Source: CAD feature listing. Evaluate the final solid. Frame: model axes, mm. Face numbers are marked on the shaded views. A direction names the side the tool comes from. Give positions to 0.01 mm unless a question says otherwise; leave off trailing zeros. Use one line per item in the form item = value. Start each with the question number.
(1) Draft query along X for the marked faces 1, 2 and 3. Return one class per face: pulls with the +X half, pulls with the -X half, needs draft (parallel to the pull), parting line crosses it, or undercut.
(2) Material intervals for line 1 along Y through (x, z) = (3, 14.25); line 2 along Z through (x, y) = (15, -34); line 3 along X through (y, z) = (2, 21), sorted ascending. Write a range as from..to.
(3) Set-up query: the marked faces 4 and 5. Return all of +Z, -Z, +X, -X, +Y, -Y with unobstructed straight access to the full face (end or side cutting, diameter ignored); none if empty.
(4) Cut plane A-A, the plane z = 3. Count the separate pieces of the cut face and the enclosed holes in it, and give its area (3 significant figures).
(5) First-contact query: P1, Ø3, axis at x = 9.88, y = -30.61, coming from the -Z side; P2, Ø12, axis at y = 15, z = 14.5, coming from the +X side; P3, Ø2, axis at y = 11, z = 13, coming from the +X side; P4, Ø2, axis at x = 5, z = 6.5, coming from the +Y side. Flat tips, straight axial feed; report the tip coordinate or a pass-through.
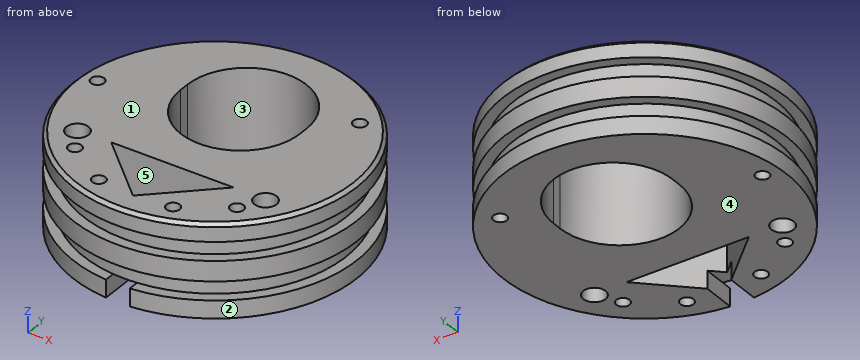
Autodesk Inventor part; units mm, degrees
ref_plane "Work Plane1" through (0, 0, 21.59) normal (0, 0, 1) x (1, 0, 0)
ref_plane "Work Plane2" through (0, 0, 6.35) normal (0, 0, -1) x (-1, 0, 0)
ref_plane "Work Plane4" through (-16.2938, -35.56, 1.651) normal (0, -1, 0) x (1, 0, 0)
sketch "Sketch1" plane through (0, 0, 0) normal (0, 0, 1) x (1, 0, 0)
  circle A0 centre (0, 0) radius 37.7444
  dimension "d0" = 75.4888
extrude "Extrusion1" add sketch "Sketch1" along normal blind 27.94
ref_plane "Work Plane1" through (0, 0, 21.59) normal (0, 0, 1) x (1, 0, 0)
sketch "Sketch2" plane through (0, 0, 21.59) normal (0, 0, 1) x (1, 0, 0)
  circle A0 centre (0, 0) radius 34.9504
  circle A1 centre (0, 0) radius 37.7444
  dimension "d4" = 2.794
extrude "Extrusion2" cut sketch "Sketch2" against normal blind 4.953
ref_plane "Work Plane2" through (0, 0, 6.35) normal (0, 0, -1) x (-1, 0, 0)
sketch "Sketch3" plane through (0, 0, 6.35) normal (0, 0, -1) x (-1, 0, 0)
  circle A0 centre (0, 0) radius 34.9504
  circle A1 centre (0, 0) radius 37.7444
  dimension "d8" = 2.794
extrude "Extrusion3" cut sketch "Sketch3" against normal blind 4.953
sketch "Sketch4" plane through (0, 0, 0) normal (0, 0, -1) x (-1, 0, 0)
  circle A0 centre (0, 0) radius 31.7754
  line L0 (-29.1271, -12.7) -> (29.1271, -12.7)
  line L1 (-19.685, -12.7) -> (-19.685, 24.9435)
  line L2 (19.685, -12.7) -> (19.685, 24.9435)
  line L3 (0, -52.8422) -> (0, 52.8422)
  circle A1 centre (0, 0) radius 37.7444
  line L4 (52.8422, 0) -> (-52.8422, 0)
  dimension "d11" = 39.37
  dimension "d12" = 5.969
  dimension "d25" = 12.7
extrude "Extrusion4" [suppressed]
sketch "Sketch5" plane through (0, 0, 27.94) normal (0, 0, 1) x (1, 0, 0)
  circle A0 centre (24.257, 20.828) radius 1.778
  circle A1 centre (-21.59, -22.86) radius 1.778
  circle A2 centre (21.59, -22.86) radius 1.778
  line L0 (0, -52.8422) -> (0, 52.8422)
  line L1 (-52.8422, 0) -> (52.8422, 0)
  circle A3 centre (-33.02, 2.54) radius 1.778
  point P0 (0, 0)
  dimension "d16" = 3.556
  dimension "d17" = 3.556
  dimension "d18" = 3.556
  dimension "d19" = 20.828
  dimension "d20" = 24.257
  dimension "d21" = 22.86
  dimension "d22" = 21.59
  dimension "d64" = 3.556
  dimension "d65" = 2.54
  dimension "d66" = 33.02
extrude "Extrusion5" cut sketch "Sketch5" against normal through all
sketch "Sketch6" plane through (0, 0, 27.94) normal (0, 0, 1) x (1, 0, 0)
  circle A0 centre (21.59, -22.86) radius 1.778
  circle A1 centre (24.257, 20.828) radius 1.778
  circle A2 centre (-21.59, -22.86) radius 1.778
  circle A3 centre (0, 0) radius 37.7444
  circle A4 centre (-21.59, -22.86) radius 1.778
  circle A5 centre (-21.59, -22.86) radius 8.255
  circle A6 centre (21.59, -22.86) radius 8.255
  line L0 (-16.3153, -16.51) -> (26.8647, -16.51)
  circle A7 centre (0, 0) radius 34.9504
  circle A8 centre (0, 0) radius 31.7754
  line L1 (0, -31.7754) -> (-16.2938, -16.51)
  line L2 (0, -31.7754) -> (16.2938, -16.51)
  dimension "d26" = 16.51
  dimension "d27" = 16.51
extrude "Extrusion6" cut sketch "Sketch6" against normal through all contours L2 L1 L0
fillet "Fillet1" [suppressed]
chamfer "Chamfer1" distance 2.54 angle 45 1 edges at (-37.7444, 0, 27.94)
sketch "Sketch9" plane through (0, 0, 27.94) normal (0, 0, 1) x (1, 0, 0)
  circle A0 centre (-9.8806, -30.607) radius 1.778
  circle A1 centre (9.8806, -30.607) radius 1.778
  line L0 (-52.8422, 0) -> (52.8422, 0)
  line L1 (0, -52.8422) -> (0, 52.8422)
  line L2 (-14.9225, -28.448) -> (14.9225, -28.448)
  line L3 (14.9225, -28.448) -> (14.9225, -34.163)
  line L4 (14.9225, -34.163) -> (-14.9225, -34.163)
  line L5 (-14.9225, -34.163) -> (-14.9225, -28.448)
  point P0 (0, 0)
  dimension "d45" = 3.556
  dimension "d46" = 3.556
  dimension "d47" = 19.7612
  dimension "d48" = 29.845
  dimension "d49" = 5.715
  dimension "d50" = 3.556
  dimension "d51" = 34.163
extrude "Extrusion9" cut sketch "Sketch9" against normal through all contours A0 | A1
sketch "Sketch11" plane through (0, 0, 0) normal (0, 0, -1) x (-1, 0, 0)
  circle A0 centre (-9.8806, -30.607) radius 1.778
  circle A1 centre (9.8806, -30.607) radius 1.778
  line L0 (16.2938, -16.51) -> (0, -31.7754)
  line L1 (0, -31.7754) -> (-16.2938, -16.51)
  line L2 (-16.2938, -16.51) -> (16.2938, -16.51)
  circle A2 centre (-21.59, -22.86) radius 1.778
  circle A3 centre (-24.257, 20.828) radius 1.778
  circle A4 centre (21.59, -22.86) radius 1.778
  circle A5 centre (0, 0) radius 37.7444
extrude "Extrusion10" cut sketch "Sketch11" against normal blind 1.651
sketch "Sketch12" plane through (0, 0, 27.94) normal (0, 0, 1) x (1, 0, 0)
  circle A0 centre (9.8806, -30.607) radius 1.778
  circle A1 centre (-9.8806, -30.607) radius 1.778
  circle A2 centre (-21.59, -22.86) radius 1.778
  circle A3 centre (24.257, 20.828) radius 1.778
  circle A4 centre (21.59, -22.86) radius 1.778
  line L0 (0, -31.7754) -> (-16.2938, -16.51)
  line L1 (-16.2938, -16.51) -> (16.2938, -16.51)
  line L2 (16.2938, -16.51) -> (0, -31.7754)
  circle A5 centre (0, 0) radius 35.2044
  circle A6 centre (0, 0) radius 37.7444
extrude "Extrusion11" cut sketch "Sketch12" against normal blind 1.651 contours A0 | A1 | A2 | A3 | A4 | L0 L1 L2 | A5 | A6
ref_plane "Work Plane4" through (-16.2938, -35.56, 1.651) normal (0, -1, 0) x (1, 0, 0)
sketch "Sketch13" plane through (-16.2938, -35.56, 1.651) normal (0, -1, 0) x (1, 0, 0)
  line L0 (16.2938, -7.239) -> (16.2938, 31.877)
  line L1 (-36.5483, -1.651) -> (69.136, -1.651)
  line L2 (8.1912, 24.638) -> (8.1912, 0)
  line L3 (54.0382, 0) -> (-21.4506, 0)
  line L4 (-21.4506, 4.699) -> (54.0382, 4.699)
  line L5 (39.6618, 24.638) -> (39.6618, 0)
  line L6 (51.2442, 4.699) -> (-18.6566, 4.699)
  line L7 (-2.049, 0) -> (34.6366, 0)
  line L8 (13.1188, 4.699) -> (19.4688, 4.699)
  line L9 (19.4688, 4.699) -> (19.4688, 0)
  line L10 (19.4688, 0) -> (13.1188, 0)
  line L11 (13.1188, 0) -> (13.1188, 4.699)
  point P0 (16.2938, -1.651)
  point P1 (13.1188, 0)
  point P2 (19.4688, 0)
  dimension "d61" = 6.35
extrude "Extrusion12" cut sketch "Sketch13" against normal mid plane 25.4 contours L3 L11 L4 L0 | L0 L4 L9 L3
sketch "Sketch14" plane through (0, 0, 1.651) normal (0, 0, -1) x (-1, 0, 0)
  circle A0 centre (-25.0506, -16.8477) radius 2.9591
  circle A1 centre (25.0506, -16.8477) radius 2.9591
  line L0 (52.8422, 0) -> (-52.8422, 0)
  line L1 (0, -52.8422) -> (0, 52.8422)
  arc A2 (3.175, -34.8059) -> (-3.175, -34.8059) centre (0, 0) ccw
  dimension "d67" = 5.9182
  dimension "d68" = 5.9182
extrude "Extrusion13" cut sketch "Sketch14" against normal through all contours A0 | A1
sketch "Sketch15" plane through (0, 0, 1.651) normal (0, 0, -1) x (-1, 0, 0)
  circle A0 centre (0, 11.0744) radius 15.875
  line L0 (0, 26.9494) -> (0, 37.7444)
  arc A1 (3.175, -37.6106) -> (-3.175, -37.6106) centre (0, 0) ccw
  dimension "d71" = 31.75
  dimension "d73" = 10.795
sketch "Sketch16" plane through (0, 0, 1.651) normal (0, 0, -1) x (-1, 0, 0)
  line L0 (0, 9.8044) -> (0, 12.3444) construction
  line L1 (15.875, 9.8044) -> (15.875, 12.3444)
  line L2 (-15.875, 12.3444) -> (-15.875, 9.8044)
  arc A0 (-15.875, 9.8044) -> (15.875, 9.8044) centre (0, 9.8044) ccw
  arc A1 (15.875, 12.3444) -> (-15.875, 12.3444) centre (0, 12.3444) ccw
  line L3 (0, -52.8422) -> (0, 52.8422)
  point P0 (0, 0)
  point P1 (0, 11.0744)
  dimension "d75" = 15.875
  dimension "d76" = 2.54
extrude "Extrusion14" cut sketch "Sketch16" against normal through all
properties part number "CameraFrontSupport"
Geometry says:
q1.face_1 = needs draft
q1.face_2 = parting line crosses it
q1.face_3 = undercut
q2.line_1 = -37.62..-28.96, -16.51..-5.78, 27.93..37.62
q2.line_2 = 1.65..6.35, 11.3..16.64, 21.59..25.98
q2.line_3 = -34.89..-34.71, -31.33..-13.82, 13.82..34.89
q3.face_4 = -Z, +X, -X, +Y, -Y
q3.face_5 = +Z, -Z
q4.separate_pieces = 1
q4.enclosed_holes = 9
q4.area = 3,190 mm^2
q5.P1 = through
q5.P2 = 36.66
q5.P3 = 36.4
q5.P4 = 37.53
